Input: dimensioned drawing with shaded views. Units: mm. Origin: part minimum x, y, z. Coordinates: 2 decimals unless noted, no trailing zeros. Write each loop counter-clockwise with the first axis right and the second up, starting at its lowest first coordinate (ties: lowest second). Pieces come first, ordered by that corner, then holes. Notation, with made-up numbers: M 3,-40 L 51,-40 A32 cw 51,-6 Z; hole C 24,-3 d5. An arc over 180 degrees is marked long. Write each question's results on one line, items separated by ' | '. Start each with the question number.
1. Ray query, probe 1 along X at (y, z) = (1.75, 11.5); probe 2 along X at (y, z) = (1.4, 12.75). Return the intervals inside material, ascending.
2. Section query A-A, the plane y = 0.95. Output: boundary loops of the cut face in (x, z).
3. Section query B-B, the plane x = 10. Output: boundary loops of the cut face in (y, z), and give its area (3 significant figures).
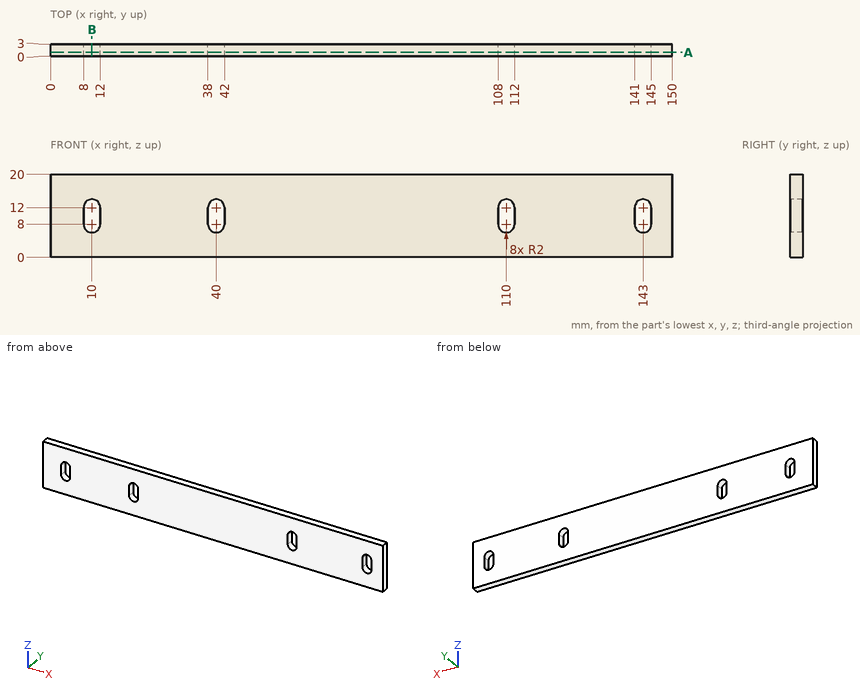
Answer:
1) probe 1: 0 to 8, 12 to 38, 42 to 108, 112 to 141, 145 to 150 | probe 2: 0 to 8.15, 11.85 to 38.15, 41.85 to 108.15, 111.85 to 141.15, 144.85 to 150
2) outline: M 0,0 L 150,0 L 150,20 L 0,20 Z; hole M 8,8 A2 ccw 12,8 L 12,12 A2 ccw 8,12 Z; hole M 38,8 A2 ccw 42,8 L 42,12 A2 ccw 38,12 Z; hole M 108,8 A2 ccw 112,8 L 112,12 A2 ccw 108,12 Z; hole M 141,8 A2 ccw 145,8 L 145,12 A2 ccw 141,12 Z
3) outline: M 0,0 L 3,0 L 3,6 L 0,6 Z; M 0,14 L 3,14 L 3,20 L 0,20 Z | area: 36.0 mm^2
